Read the model definition and answer for the solid it produces. Units are mm, in the model's axes. A direction names the side the tool comes from. Give positions to 0.01 mm unless a question says otherwise; leave off trailing zeros. Write each loop counter-clockwise with the first axis right and the second up, starting at its lowest first coordinate (ties: lowest second). Pieces come first, ordered by that corner, then holes. Notation, with made-up numbers: (52, 50.5) -> (60, 50.5) arc R5 cw to (60, 59.5) -> close; hole circle Ø8 at (-9.5, 40.5). An arc over 180 degrees is marked (long way). Answer as CSV lines item,"result". Start each with the question number.
1. A tool of negligible diameter and unlimited length cuts with its end or side. For faces 5 (the flat face through (-2, 6, 6)), 6 (the flat face through (-2, 6, 15)), 7 (the cylindrical face through (16.974, 8.425, 17.288)), from which of +Z, -Z, +X, -X, +Y, -Y can it reach the whole face along a straight path? Write none if from no direction.
2. The part is cut by section A-A, the plane y = 0. Give the number of separate pieces and of enclosed holes in the cut face, and give its area (4 significant figures).
3. The part is cut by section C-C, the plane y = -18. Determine the outline of the cut face in (x, z).
4. Given pin 1 (5 mm diameter, centred on y = 17, z = 15.5, fed in from -X); pin 2 (4 mm diameter, centred on x = 15.59, y = 9, fed in from -Z); pin 3 (1.9 mm diameter, centred on x = 15.5, y = -9.5, fed in from +Z), each flat-ended and moving along its own axis, determine where each tip first touches the part or whether it passes through.
5. The part is cut by section D-D, the plane y = 9. Determine the outline of the cut face in (x, z), and give its area (3 significant figures).
6. For a pull along X with two mould halves and no side action, classify faces 1 (the cylindrical face through (-10.382, -19.961, 12.951)), 2 (the cylindrical face through (-17.537, -8.914, 18.028)), 3 (the cylindrical face through (-19.48, 0.61, 14.82)), 4 (the flat face through (-11.7, 19.4, 16.5)) as pulls with the +X half, pulls with the -X half, needs draft (parallel to the pull), parting line crosses it, or undercut.
7. Find the intervals of material crossed by line 1 (Z direction, x = 2.5, y = 18); line 2 (Z direction, x = -15, y = 18); line 3 (Y direction, x = 9, z = 13.75), in increasing order.
from build123d import *

# Parameters (mm, degrees)
SKETCH1_R           = 25
BOSS_EXTRUDE1_DEPTH = 20
SKETCH2_R           = 1.95
CUT_EXTRUDE1_DEPTH  = 4
SKETCH4_R           = 1.5
CUT_EXTRUDE2_DEPTH  = 21
SKETCH6_R           = 7.9
CUT_EXTRUDE3_DEPTH  = 21
BOSS_EXTRUDE4_START = -6
SKETCH7_R           = 7.9
SKETCH7_R_2         = 6
BOSS_EXTRUDE4_DEPTH = 9
SKETCH9_R           = 26
SKETCH9_R_2         = 25
BOSS_EXTRUDE6_DEPTH = 3.5
SKETCH10_R          = 25
SKETCH10_R_2        = 22.5
CUT_EXTRUDE5_DEPTH  = 16.5
SKETCH11_R          = 22.5
SKETCH11_R_2        = 12.5
CUT_EXTRUDE6_DEPTH  = 9.5
SKETCH12_R          = 3
CUT_EXTRUDE7_DEPTH  = 5
CIRPATTERN2_COUNT   = 3
SKETCH13_R          = 1.6
CUT_EXTRUDE8_DEPTH  = 21
CIRPATTERN3_COUNT   = 6
SKETCH15_R          = 12.5
SKETCH15_R_2        = 7.9
BOSS_EXTRUDE7_DEPTH = 5


with BuildPart() as part:
    # Sketch1 → Boss-Extrude1 (new body)
    with BuildSketch(Plane.XY):
        Circle(SKETCH1_R)
    extrude(amount=BOSS_EXTRUDE1_DEPTH)

    # Sketch2 → Cut-Extrude1 (cut)
    with BuildSketch(Plane.XY.offset(20)):
        with Locations((0, 18)):
            Circle(SKETCH2_R)
        with Locations((15.588457268, -9)):
            Circle(SKETCH2_R)
        with Locations((-15.588457268, -9)):
            Circle(SKETCH2_R)
    extrude(amount=-CUT_EXTRUDE1_DEPTH, mode=Mode.SUBTRACT)

    # Sketch4 → Cut-Extrude2 (cut, through all)
    with BuildSketch(Plane.XY.offset(20)):
        with Locations((15.588457268, 9)):
            Circle(SKETCH4_R)
        with Locations((0, -18)):
            Circle(SKETCH4_R)
        with Locations((-15.588457268, 9)):
            Circle(SKETCH4_R)
    extrude(amount=-CUT_EXTRUDE2_DEPTH, mode=Mode.SUBTRACT)

    # Sketch6 → Cut-Extrude3 (cut, through all)
    with BuildSketch(Plane.XY.offset(20)):
        Circle(SKETCH6_R)
    extrude(amount=-CUT_EXTRUDE3_DEPTH, mode=Mode.SUBTRACT)

    # Sketch7 → Boss-Extrude4 (add)
    with BuildSketch(Plane(origin=(0, 0, 0), x_dir=(-1, 0, 0), z_dir=(0, 0, -1)).offset(BOSS_EXTRUDE4_START)):
        Circle(SKETCH7_R)
        Circle(SKETCH7_R_2, mode=Mode.SUBTRACT)
    extrude(amount=-BOSS_EXTRUDE4_DEPTH)

    # Sketch9 → Boss-Extrude6 (add)
    with BuildSketch(Plane.XY.offset(20)):
        Circle(SKETCH9_R)
        Circle(SKETCH9_R_2, mode=Mode.SUBTRACT)
    extrude(amount=-BOSS_EXTRUDE6_DEPTH)

    # Sketch10 → Cut-Extrude5 (cut)
    with BuildSketch(Plane(origin=(0, 0, 0), x_dir=(-1, 0, 0), z_dir=(0, 0, -1))):
        Circle(SKETCH10_R)
        Circle(SKETCH10_R_2, mode=Mode.SUBTRACT)
    extrude(amount=-CUT_EXTRUDE5_DEPTH, mode=Mode.SUBTRACT)

    # Sketch11 → Cut-Extrude6 (cut)
    with BuildSketch(Plane(origin=(0, 0, 0), x_dir=(-1, 0, 0), z_dir=(0, 0, -1))):
        Circle(SKETCH11_R)
        Circle(SKETCH11_R_2, mode=Mode.SUBTRACT)
    extrude(amount=-CUT_EXTRUDE6_DEPTH, mode=Mode.SUBTRACT)

    # Sketch12 → Cut-Extrude7 (cut)
    with BuildSketch(Plane(origin=(0, 0, 9.5), x_dir=(-1, 0, 0), z_dir=(0, 0, -1))):
        with Locations((-15.588457268, 9)):
            Circle(SKETCH12_R)
    cut_extrude7 = extrude(amount=-CUT_EXTRUDE7_DEPTH, mode=Mode.SUBTRACT)

    # CirPattern2: Cut-Extrude7 ×3 about axis
    cirpattern2_axis = Axis((0, 0, 0), (0, 0, 1))
    for i in range(1, CIRPATTERN2_COUNT):
        add(cut_extrude7.rotate(cirpattern2_axis, i * 360 / CIRPATTERN2_COUNT), mode=Mode.SUBTRACT)

    # Sketch13 → Cut-Extrude8 (cut, through all)
    with BuildSketch(Plane.XY.offset(20)):
        with Locations((-9, 15.588457268)):
            Circle(SKETCH13_R)
    cut_extrude8 = extrude(amount=-CUT_EXTRUDE8_DEPTH, mode=Mode.SUBTRACT)

    # CirPattern3: Cut-Extrude8 ×6 about axis
    cirpattern3_axis = Axis((0, 0, 0), (0, 0, 1))
    for i in range(1, CIRPATTERN3_COUNT):
        add(cut_extrude8.rotate(cirpattern3_axis, i * 360 / CIRPATTERN3_COUNT), mode=Mode.SUBTRACT)

    # Sketch15 → Boss-Extrude7 (add)
    with BuildSketch(Plane(origin=(0, 0, 0), x_dir=(-1, 0, 0), z_dir=(0, 0, -1))):
        Circle(SKETCH15_R)
        Circle(SKETCH15_R_2, mode=Mode.SUBTRACT)
    extrude(amount=BOSS_EXTRUDE7_DEPTH)


solid = part.part
Results found:
1,face 5,"-Z"
1,face 6,"+Z"
1,face 7,"+Z, -Z"
2,separate pieces,"4"
2,enclosed holes,"0"
2,area,"431.5 mm²"
3,outline,"(-18.76, 16.5) -> (-13.5, 16.5) -> (-13.5, 9.5) -> (-3, 9.5) -> (-3, 14.5) -> (-1.5, 14.5) -> (-1.5, 20) -> (-18.76, 20) -> close; (1.5, 14.5) -> (3, 14.5) -> (3, 9.5) -> (13.5, 9.5) -> (13.5, 16.5) -> (18.76, 16.5) -> (18.76, 20) -> (1.5, 20) -> close"
4,pin 1,"stops at x = -21.44"
4,pin 2,"stops at z = 14.5"
4,pin 3,"stops at z = 16"
5,outline,"(-24.39, 16.5) -> (-20.62, 16.5) -> (-20.62, 9.5) -> (-18.59, 9.5) -> (-18.59, 14.5) -> (-17.09, 14.5) -> (-17.09, 20) -> (-24.39, 20) -> close; (-14.09, 14.5) -> (-12.59, 14.5) -> (-12.59, 9.5) -> (-8.67, 9.5) -> (-8.67, -5) -> (8.67, -5) -> (8.67, 9.5) -> (12.59, 9.5) -> (12.59, 14.5) -> (14.09, 14.5) -> (14.09, 20) -> (-14.09, 20) -> close; (17.09, 14.5) -> (18.59, 14.5) -> (18.59, 9.5) -> (20.62, 9.5) -> (20.62, 16.5) -> (24.39, 16.5) -> (24.39, 20) -> (17.09, 20) -> close"
5,area,"618 mm²"
6,face 1,"parting line crosses it"
6,face 2,"undercut"
6,face 3,"undercut"
6,face 4,"needs draft"
7,line 1,"z = 9.5 to 20"
7,line 2,"z = 16.5 to 20"
7,line 3,"y = -20.62 to -17.19, -13.99 to 13.99, 17.19 to 20.62"
